Can you work these out from the model? Positions are in its coordinate system, mm. A direction names the side the tool comes from. Coordinates: 2 decimals unless noted, no trailing zeros. Loops run counter-clockwise (first coordinate to the right, second up) from the corner with the lowest first, then second, coordinate; pieces in that order, holes last. Notation, with made-up numbers: M 79,-20.5 L 93,-20.5 A28 cw 93,17.5 Z; hole C 51,76 d3. An arc over 180 degrees is marked long. Return JSON: item names as keys, results as strings. Group by question number.
```python
from build123d import *

# Parameters (mm, degrees)
SKETCH1_R           = 28.1
BOSS_EXTRUDE1_DEPTH = 1
SKETCH2_R           = 18.6
CUT_EXTRUDE1_DEPTH  = 58.8
SKETCH3_W           = 222.683092022
SKETCH3_H           = 364.2827524
BOSS_EXTRUDE2_DEPTH = 58.8
SKETCH4_W           = 207.917403516
SKETCH4_H           = 348.54429772
CUT_EXTRUDE2_DEPTH  = 55.8
SKETCH9_R           = 3
CUT_EXTRUDE8_DEPTH  = 10
SKETCH10_R          = 3.75
CUT_EXTRUDE9_DEPTH  = 10
CUT_EXTRUDE14_DEPTH = 500
SKETCH6_R           = 3.75
CUT_EXTRUDE5_DEPTH  = 400
SKETCH8_R           = 10
CUT_EXTRUDE7_DEPTH  = 10


with BuildPart() as part:
    # Sketch1 → Boss-Extrude1 (new body)
    with BuildSketch(Plane(origin=(0, 0, 0), x_dir=(1, 0, 0), z_dir=(0, 1, 0))):
        Circle(SKETCH1_R)
    extrude(amount=BOSS_EXTRUDE1_DEPTH)

    # Sketch2 → Cut-Extrude1 (cut)
    with BuildSketch(Plane(origin=(0, 1, 0), x_dir=(1, 0, 0), z_dir=(0, 1, 0))):
        with Locations((0, -7)):
            Circle(SKETCH2_R)
    extrude(amount=-CUT_EXTRUDE1_DEPTH, mode=Mode.SUBTRACT)

    # Sketch3 → Boss-Extrude2 (add)
    with BuildSketch(Plane(origin=(0, 0, 0), x_dir=(-1, 0, 0), z_dir=(0, -1, 0))):
        Rectangle(SKETCH3_W, SKETCH3_H)
    extrude(amount=BOSS_EXTRUDE2_DEPTH)

    # Sketch4 → Cut-Extrude2 (cut)
    with BuildSketch(Plane(origin=(0, -58.8, 0), x_dir=(-1, 0, 0), z_dir=(0, -1, 0))):
        Rectangle(SKETCH4_W, SKETCH4_H)
    extrude(amount=-CUT_EXTRUDE2_DEPTH, mode=Mode.SUBTRACT)

    # Sketch9 → Cut-Extrude8 (cut)
    with BuildSketch(Plane(origin=(0, 0, 0), x_dir=(1, 0, 0), z_dir=(0, 1, 0))):
        with Locations((0, -7)):
            Circle(SKETCH9_R)
    extrude(amount=-CUT_EXTRUDE8_DEPTH, mode=Mode.SUBTRACT)

    # Sketch10 → Cut-Extrude9 (cut)
    with BuildSketch(Plane(origin=(0, 1, 0), x_dir=(1, 0, 0), z_dir=(0, 1, 0))):
        with Locations((0, 19.85)):
            Circle(SKETCH10_R)
    extrude(amount=-CUT_EXTRUDE9_DEPTH, mode=Mode.SUBTRACT)

    # Sketch11 → Cut-Extrude14 (cut)
    with BuildSketch(Plane(origin=(0, -58.8, 0), x_dir=(-1, 0, 0), z_dir=(0, -1, 0))):
        Polygon((38.658453989, -17.8586238), (-111.341546011, -17.8586238), (-111.341546011, 182.1413762), (111.341546011, 182.1413762), (111.341546011, -182.1413762), (38.658453989, -182.1413762), align=None)
    extrude(amount=-CUT_EXTRUDE14_DEPTH, mode=Mode.SUBTRACT)

    # Sketch6 → Cut-Extrude5 (cut)
    with BuildSketch(Plane(origin=(0, 1, 0), x_dir=(1, 0, 0), z_dir=(0, 1, 0))):
        with Locations((0, 18.75)):
            Circle(SKETCH6_R)
    extrude(amount=-CUT_EXTRUDE5_DEPTH, mode=Mode.SUBTRACT)

    # Sketch8 → Cut-Extrude7 (cut)
    with BuildSketch(Plane(origin=(0, 0, -182.1413762), x_dir=(-1, 0, 0), z_dir=(0, 0, -1))):
        with Locations((-86.573671766, -25.011155335)):
            Circle(SKETCH8_R)
    extrude(amount=-CUT_EXTRUDE7_DEPTH, mode=Mode.SUBTRACT)


solid = part.part
```
1) Suppose I cut it at C-C, the plane x = -2.5. List the corners of the cut face in (y, z) for me, then the cut area to 3 significant figures.
2) If I drill on line 1 (X direction, y = -22, z = 80.5); line 2 (Y direction, x = 95.5, z = 172); line 3 (Z direction, x = 10, y = -36), over which ranges is the centre line in solid material (lowest first)? Write a range as from..to.
3) Suppose I cut it at B-B, the plane y = -8. List the corners of the cut face in (x, z) for me, then the cut area to 3 significant figures.
4) For faces 1 (the face through (-0.2, 0.5, 25.6)), 2 (the face through (37, -29, 182.141)), 3 (the face through (34, -31, 174.272)), which set-ups out of +Z, -Z, +X, -X, +Y, -Y let a thin tool reach every point of the face, with its end or its side?
5) For pin 1 (1 mm diameter, centred on y = -13.5, z = 82.5, fed in from -X); pin 2 (8 mm diameter, centred on x = 92, y = -51.5, fed in from -Z); pin 3 (2.5 mm diameter, centred on x = -3, z = 20.5, fed in from +Y), each with a flat end and sliding along its axis, tell me the tip position at first contact or that it passes through.
6) Suppose I cut it at A-A, the plane x = 91. List the corners of the cut face in (y, z) for me, then the cut area to 3 significant figures.
7) If we mould it in two halves opening along X, with no side actions, what happens to faces 4 (the face through (-38.658, -1, 137)), 5 (the face through (34, -3, 95)), 6 (the face through (-0.3, 0.5, 28.1)), 7 (the face through (0, 0, 21))? For each: +X half, -X half, draft (parallel to the pull), parting line (faces both ways), or undercut.
Returned:
{
 "1": {"outline": "M -58.8,174.27 L -3,174.27 L -3,17.86 L 0,17.86 L 0,25.43 L 1,25.43 L 1,27.99 L 0,27.99 L 0,182.14 L -58.8,182.14 Z", "area": "935 mm²"},
 "2": {"line 1": "x = 103.96..111.34", "line 2": "y = -3..0", "line 3": "z = 174.27..182.14"},
 "3": {"outline": "M -38.66,174.27 L 103.96,174.27 L 103.96,17.86 L 111.34,17.86 L 111.34,182.14 L -38.66,182.14 Z", "area": "2,340 mm²"},
 "4": {"face 1": "-Z, +Y", "face 2": "+Z, +X, -X, +Y, -Y", "face 3": "-Z, -X, -Y"},
 "5": {"pin 1": "stops at x = 103.96", "pin 2": "stops at z = 174.27", "pin 3": "stops at y = 0"},
 "6": {"outline": "M -58.8,174.27 L -3,174.27 L -3,17.86 L 0,17.86 L 0,182.14 L -58.8,182.14 Z", "area": "932 mm²"},
 "7": {"face 4": "-X half", "face 5": "draft", "face 6": "parting line", "face 7": "undercut"}
}
